Read the model definition and answer for the solid it produces. Units are mm, in the model's axes. Face numbers are marked on the shaded views. A direction names the side the tool comes from. Coordinates: 2 decimals unless noted, no trailing zeros. Loops run counter-clockwise (first coordinate to the right, second up) from the corner with the lowest first, then second, coordinate; pieces in that order, holes last.
Q1. Section C-C (z = 7.5) is taken. Give the vertices of the cut face in (x, y), then the cut area to 3 significant figures.
Q2. A flat-ended cylindrical pin translates along its axis: P1, Ø4, axis at x = 35.5, z = 21, coming from the +Y side. Find the tip coordinate at first contact, or state that the pin passes through.
Q3. Section A-A (y = 13.5) is taken. Give the vertices of the cut face in (x, z), then the cut area to 3 significant figures.
Q4. Section B-B (x = 44) is taken. Give the vertices of the cut face in (y, z), then the cut area to 3 significant figures.
Q5. Straight lines are drawn through the part: line 1 (X direction, y = 8.25, z = 31); line 2 (Z direction, x = 27.5, y = 22.5); line 3 (Y direction, x = 8.5, z = 2). For each, find the intervals that lie inside material, in ascending order.
Q6. Which of the six approach directions +Z, -Z, +X, -X, +Y, -Y give full straight-line access (tool end or side, diameter ignored) to the marked faces 1, 2 and 3?
Q7. The mould has two halves that part along Z. Classify the marked faces 4, 5 and 6: pulls with the +Z half, pulls with the -Z half, needs draft (parallel to the pull), parting line crosses it, or undercut.
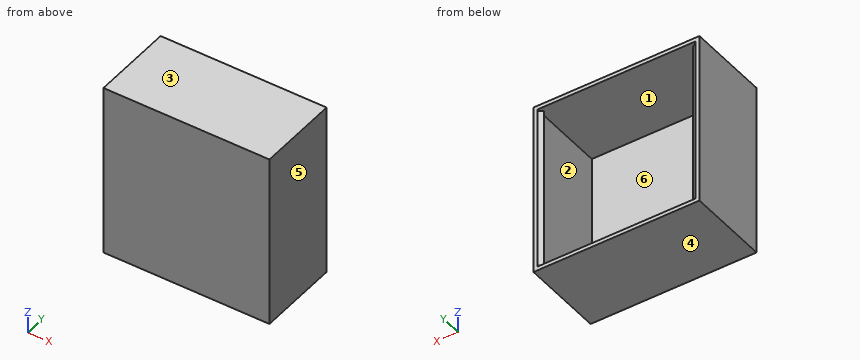
Autodesk Inventor part; units mm, degrees
ref_plane "YZ Plane" through (0, 0, 0) normal (1, 0, 0) x (0, 1, 0)
ref_plane "XZ Plane" through (0, 0, 0) normal (0, 1, 0) x (-1, 0, 0)
ref_plane "XY Plane" through (0, 0, 0) normal (0, 0, 1) x (1, 0, 0)
sketch "Sketch1" plane through (0, 0, 0) normal (0, 0, 1) x (1, 0, 0)
  line L0 (0, 0) -> (50.8, 0)
  line L1 (50.8, 0) -> (50.8, 25.4)
  line L2 (0, 25.4) -> (0, 0)
  line L3 (1.2, 1.2) -> (49.6, 1.2)
  line L4 (49.6, 1.2) -> (49.6, 23.4)
  line L5 (1.2, 23.4) -> (1.2, 1.2)
  line L6 (50.8, 25.4) -> (49.6, 25.4)
  line L7 (1.2, 25.4) -> (0, 25.4)
  line L8 (2.614, 24.4) -> (1.2, 23.4)
  line L9 (1.2, 25.4) -> (2.614, 24.4)
  line L10 (48.186, 24.4) -> (49.6, 25.4)
  line L11 (48.186, 24.4) -> (49.6, 23.4)
  line L12 (1.2, 25.4) -> (1.2, 23.4) construction
  line L13 (1.2, 24.4) -> (2.614, 24.4) construction
  line L14 (49.6, 23.4) -> (49.6, 25.4) construction
  line L15 (49.6, 24.4) -> (48.186, 24.4) construction
  dimension "Width" = 50.8
  dimension "Height" = 25.4
  dimension "Offset" = 1.2
  dimension "LeftEdge" = 1.2
  dimension "RightEdge" = 1.2
  dimension "LT_Height" = 2
  dimension "LT_Width" = 1.414
  dimension "RT_Width" = 1.414
  dimension "RT_Height" = 2
extrude "Extrusion1" add sketch "Sketch1" along normal blind 50
sketch "Sketch2" plane through (0, 0, 50) normal (0, 0, 1) x (1, 0, 0)
  line L0 (0, 25.4) -> (0, 0)
  line L1 (0, 0) -> (50.8, 0)
  line L2 (50.8, 0) -> (50.8, 25.4)
  line L3 (50.8, 25.4) -> (49.6, 25.4)
  line L4 (49.6, 25.4) -> (48.186, 24.4)
  line L5 (48.186, 24.4) -> (49.6, 23.4)
  line L6 (49.6, 23.4) -> (49.6, 1.2)
  line L7 (49.6, 1.2) -> (1.2, 1.2)
  line L8 (1.2, 1.2) -> (1.2, 23.4)
  line L9 (1.2, 23.4) -> (2.614, 24.4)
  line L10 (2.614, 24.4) -> (1.2, 25.4)
  line L11 (1.2, 25.4) -> (0, 25.4)
  line L12 (1.2, 23.4) -> (1.2, 25.4)
  line L13 (1.2, 1.2) -> (1.2, 23.4)
  line L14 (49.6, 23.4) -> (49.6, 25.4)
extrude "Extrusion2" add sketch "Sketch2" along normal blind 0.4 contours L11 L12 L8 L7 L6 L14 L3 L2 L1 L0
sketch "Sketch3" plane through (0, 0, 50.4) normal (0, 0, 1) x (1, 0, 0)
  line L0 (50.8, 0) -> (50.8, 25.4)
  line L1 (0, 0) -> (50.8, 0)
  line L2 (50.8, 0) -> (50.8, 25.4)
  line L3 (50.8, 25.4) -> (0, 25.4)
  line L4 (0, 25.4) -> (0, 0)
ref_plane "Work Plane1" through (0, 0, 25) normal (0, 0, 1) x (1, 0, 0)
extrude "Extrusion3" add sketch "Sketch3" along normal blind 1.2
mirror "Mirror1" about plane through (0, 0, 25) normal (0, 0, 1) of "Extrusion3", "Extrusion2"
equation "\"LeftEdge\" = Offset"
equation "\"RightEdge\" = Offset"
equation "\"RT_Width\" = LT_Width"
equation "\"RT_Height\" = LT_Height"
properties part number "channel_base"
Numbers:
1. outline: (0, 0) - (50.8, 0) - (50.8, 25.4) - (49.6, 25.4) - (48.19, 24.4) - (49.6, 23.4) - (49.6, 1.2) - (1.2, 1.2) - (1.2, 23.4) - (2.61, 24.4) - (1.2, 25.4) - (0, 25.4) - close
1. area: 122 mm2
2. P1: stops at y = 1.2
3. outline: (0, -1.6) - (50.8, -1.6) - (50.8, 51.6) - (0, 51.6) - close; hole (1.2, -0.4) - (49.6, -0.4) - (49.6, 50.4) - (1.2, 50.4) - close
3. area: 244 mm2
4. outline: (0, -1.6) - (25.4, -1.6) - (25.4, -0.4) - (1.2, -0.4) - (1.2, 50.4) - (25.4, 50.4) - (25.4, 51.6) - (0, 51.6) - close
4. area: 122 mm2
5. line 1: x = 0 to 1.2, 49.6 to 50.8
5. line 2: z = -1.6 to -0.4, 50.4 to 51.6
5. line 3: y = 0 to 1.2
6. face 1: +Y
6. face 2: none
6. face 3: +Z, +X, -X, +Y, -Y
7. face 4: pulls with the -Z half
7. face 5: needs draft
7. face 6: undercut
